from build123d import *

# Parameters (mm, degrees)
SKETCH1_W           = 101.6
SKETCH1_H           = 76.2
BOSS_EXTRUDE1_DEPTH = 101.6
SKETCH3_W           = 76.2
SKETCH3_H           = 76.2
CUT_EXTRUDE1_DEPTH  = 76.2
SKETCH4_R           = 25.4
BOSS_EXTRUDE2_DEPTH = 50.8
SKETCH5_W           = 76.2
SKETCH5_H           = 76.2
BOSS_EXTRUDE3_DEPTH = 76.2
SKETCH6_R           = 12.7
CUT_EXTRUDE2_DEPTH  = 262.509005581
CUT_EXTRUDE3_REACH  = 263.509
SKETCH7_R           = 12.7


with BuildPart() as part:
    # Sketch1 → Boss-Extrude1 (new body)
    with BuildSketch(Plane(origin=(0, 0, 0), x_dir=(1, 0, 0), z_dir=(0, 1, 0))):
        with Locations((50.8, 38.1)):
            Rectangle(SKETCH1_W, SKETCH1_H)
    extrude(amount=BOSS_EXTRUDE1_DEPTH)

    # Sketch3 → Cut-Extrude1 (cut)
    with BuildSketch(Plane.XZ):
        with Locations((50.8, -38.1)):
            Rectangle(SKETCH3_W, SKETCH3_H)
    extrude(amount=-CUT_EXTRUDE1_DEPTH, mode=Mode.SUBTRACT)

    # Sketch4 → Boss-Extrude2 (add)
    with BuildSketch(Plane(origin=(0, 101.6, 0), x_dir=(1, 0, 0), z_dir=(0, 1, 0))):
        with Locations(Location((50.8, 38.1, 0), (0, 0, 270))):
            Circle(SKETCH4_R)
    extrude(amount=BOSS_EXTRUDE2_DEPTH)

    # Sketch5 → Boss-Extrude3 (add)
    with BuildSketch(Plane(origin=(0, 152.4, 0), x_dir=(1, 0, 0), z_dir=(0, 1, 0))):
        with Locations((50.8, 38.1)):
            Rectangle(SKETCH5_W, SKETCH5_H)
    extrude(amount=BOSS_EXTRUDE3_DEPTH)

    # Sketch6 → Cut-Extrude2 (cut, through all)
    with BuildSketch(Plane(origin=(101.6, 0, 0), x_dir=(0, 0, -1), z_dir=(1, 0, 0))):
        with Locations((38.1, 25.4)):
            Circle(SKETCH6_R)
    extrude(amount=-CUT_EXTRUDE2_DEPTH, mode=Mode.SUBTRACT)

    # Sketch7 → Cut-Extrude3 (cut, up to next)
    with BuildSketch(Plane(origin=(0, 0, -76.2), x_dir=(-1, 0, 0), z_dir=(0, 0, -1)), mode=Mode.PRIVATE) as cut_extrude3_sk1:
        with Locations((-50.8, 203.2)):
            Circle(SKETCH7_R)
    cut_extrude3_tool1 = extrude(cut_extrude3_sk1.sketch, amount=-CUT_EXTRUDE3_REACH, mode=Mode.PRIVATE) & part.part
    add(cut_extrude3_tool1.solids().sort_by_distance((50.8, 203.2, -76.2))[0], mode=Mode.SUBTRACT)


solid = part.part
Work out the finished part from the listing and answer in its coordinate system (mm). A direction names the side the tool comes from. Give positions to 0.01 mm unless a question says otherwise; leave off trailing zeros. Loops run counter-clockwise (first coordinate to the right, second up) from the corner with the lowest first, then second, coordinate; pieces in that order, holes last. Notation, with made-up numbers: (-10, 49) - (5, 49) arc R11 cw to (5, 64) - close; hole circle Ø1 at (-33, 51). An arc over 180 degrees is marked (long way). Answer in a Markdown table with one row per item. Add a question column.
Q1. Consider line 1 along X through (y, z) = (73.5, -38); line 2 along Z through (x, y) = (3, 25); line 3 along Y through (x, z) = (9.25, -38.1). Determine where each line is inside the solid, lowest interval first.
Q2. A tool of negligible diameter and unlimited length cuts with its end or side. For faces 4 (the flat face through (88.9, 46, -39)), 5 (the flat face through (12.7, 190, -38)), 6 (the flat face through (50, 190, -76.2)), 7 (the flat face through (50, 101.6, -64)), 8 (the flat face through (88.9, 190, -38)), from which of +Z, -Z, +X, -X, +Y, -Y can it reach the whole face along a straight path? Write none if from no direction.
Q3. The part is cut by section D-D (x = 18.5). Determine the outline of the cut face in (y, z), and give its area (3 significant figures).
Q4. The part is cut by section C-C (z = -69). Determine the outline of the cut face in (x, y), and give its area (3 significant figures).
Q5. The part is cut by section A-A (z = -38.1). Determine the outline of the cut face in (x, y), and give its area (3 significant figures).
Q6. Each of these flat-tipped pins is pushed along its axis until it touches: P1, Ø1.5, axis at y = 120, z = -47, coming from the -X side; P2, Ø1.5, axis at x = 64.5, z = -30.5, coming from the -Y side; P3, Ø4, axis at y = 174, z = -48.5, coming from the -X side. Where does it stop, or does it pass through?
Q7. The part is cut by section B-B (y = 63.5). Determine the outline of the cut face in (x, z), and give its area (3 significant figures).
Q8. Determine the mould class of faces 1 (the flat face through (6, 0, -39)), 2 (the cylindrical face through (95.339, 36.109, -44.927)), 3 (the cylindrical face through (72.22, 126.64, -24.45)) for opening direction Z: released by +Z, released by -Z, zero draft, split by the parting line, or undercut.
Solution:
| question | item | result |
|---|---|---|
| 1 | line 1 | x = 0 to 12.7, 88.9 to 101.6 |
| 1 | line 2 | z = -76.2 to -50.79, -25.41 to 0 |
| 1 | line 3 | y = 0 to 12.7, 38.1 to 101.6 |
| 2 | face 4 | +Z, -Z, -Y |
| 2 | face 5 | +Z, -Z, -X, +Y |
| 2 | face 6 | -Z, +X, -X, +Y, -Y |
| 2 | face 7 | none |
| 2 | face 8 | +Z, -Z, +X, +Y |
| 3 | outline | (76.2, -76.2) - (101.6, -76.2) - (101.6, 0) - (76.2, 0) - close; (152.4, -76.2) - (228.6, -76.2) - (228.6, 0) - (152.4, 0) - close |
| 3 | area | 7,740 mm² |
| 4 | outline | (0, 0) - (12.7, 0) - (12.7, 76.2) - (88.9, 76.2) - (88.9, 0) - (101.6, 0) - (101.6, 101.6) - (0, 101.6) - close; (12.7, 152.4) - (88.9, 152.4) - (88.9, 228.6) - (12.7, 228.6) - close; hole circle Ø25.4 at (50.8, 203.2) |
| 4 | area | 9,820 mm² |
| 5 | outline | (0, 0) - (12.7, 0) - (12.7, 12.7) - (0, 12.7) - close; (0, 38.1) - (12.7, 38.1) - (12.7, 76.2) - (88.9, 76.2) - (88.9, 38.1) - (101.6, 38.1) - (101.6, 101.6) - (76.2, 101.6) - (76.2, 152.4) - (88.9, 152.4) - (88.9, 228.6) - (12.7, 228.6) - (12.7, 152.4) - (25.4, 152.4) - (25.4, 101.6) - (0, 101.6) - close; (88.9, 0) - (101.6, 0) - (101.6, 12.7) - (88.9, 12.7) - close; hole circle Ø25.4 at (50.8, 203.2) |
| 5 | area | 11,800 mm² |
| 6 | P1 | stops at x = 26.74 |
| 6 | P2 | stops at y = 76.2 |
| 6 | P3 | stops at x = 12.7 |
| 7 | outline | (0, -76.2) - (12.7, -76.2) - (12.7, 0) - (0, 0) - close; (88.9, -76.2) - (101.6, -76.2) - (101.6, 0) - (88.9, 0) - close |
| 7 | area | 1,940 mm² |
| 8 | face 1 | zero draft |
| 8 | face 2 | undercut |
| 8 | face 3 | split by the parting line |
